Read the model definition and answer for the solid it produces. Units are mm, in the model's axes. Face numbers are marked on the shaded views. Coordinates: 2 decimals unless noted, no trailing zeros. Order: outer loops, then holes, each group sorted by start corner. A loop starts at its lowest first (then second) coordinate and runs counter-clockwise, first axis right, second up. Notation, with made-up numbers: (-31, 59.25) -> (-9, 59.25) arc R14 cw to (-9, 82.25) -> close; hole circle Ø8 at (49.5, 6). An arc over 180 degrees is marked (long way). Answer in a Markdown table with one row per item.
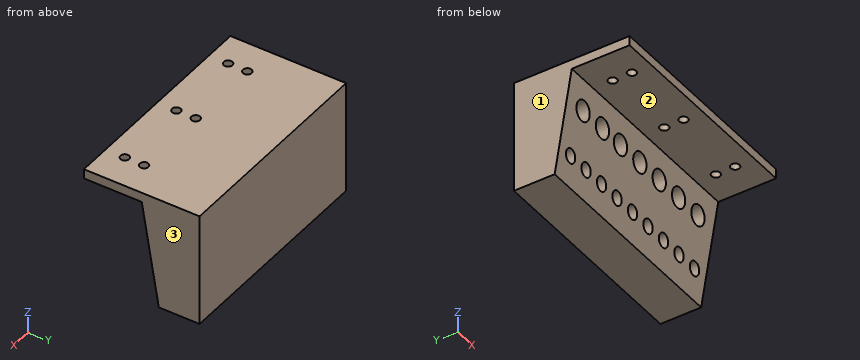
from build123d import *

# Parameters (mm, degrees)
F1_DEPTH = 25
F2_W     = 113.5
F2_H     = 53.5
F3_DEPTH = 5
F5_DEPTH = 133.9
F6_W     = 113.5
F6_H     = 60
F7_DEPTH = 5
F9_DEPTH = 25


with BuildPart() as f1:
    # F0 (on Front) → F1 (new body)
    with BuildSketch(Plane.XZ):
        with BuildLine():
            Line((30.7684078276, 51.75), (-82.7315921724, 51.75))
            Line((-82.7315921724, 51.75), (-82.7315921724, 37.7107225358))
            Line((-82.7315921724, 37.7107225358), (-75.4815921724, 37.7107225358))
            ThreePointArc((-75.4815921724, 37.7107225358), (-70.4815921724, 42.7107225358), (-65.4815921724, 37.7107225358))
            Line((-65.4815921724, 37.7107225358), (-60.4815921724, 37.7107225358))
            ThreePointArc((-60.4815921724, 37.7107225358), (-55.4815921724, 42.7107225358), (-50.4815921724, 37.7107225358))
            Line((-50.4815921724, 37.7107225358), (-46.4815921724, 37.7107225358))
            ThreePointArc((-46.4815921724, 37.7107225358), (-41.4815921724, 42.7107225358), (-36.4815921724, 37.7107225358))
            Line((-36.4815921724, 37.7107225358), (-31.4815921724, 37.7107225358))
            ThreePointArc((-31.4815921724, 37.7107225358), (-26.4815921724, 42.7107225358), (-21.4815921724, 37.7107225358))
            Line((-21.4815921724, 37.7107225358), (-16.4815921724, 37.7107225358))
            ThreePointArc((-16.4815921724, 37.7107225358), (-11.4815921724, 42.7107225358), (-6.4815921724, 37.7107225358))
            Line((-6.4815921724, 37.7107225358), (-1.4815921724, 37.7107225358))
            ThreePointArc((-1.4815921724, 37.7107225358), (3.5184078276, 42.7107225358), (8.5184078276, 37.7107225358))
            Line((8.5184078276, 37.7107225358), (13.5184078276, 37.7107225358))
            ThreePointArc((13.5184078276, 37.7107225358), (18.5184078276, 42.7107225358), (23.5184078276, 37.7107225358))
            Line((23.5184078276, 37.7107225358), (30.7684078276, 37.7107225358))
            Line((30.7684078276, 37.7107225358), (30.7684078276, 51.75))
        make_face()
        with BuildLine():
            Line((-77.4815921724, 12.7484267578), (-82.7315921724, 12.7484267578))
            Line((-82.7315921724, 12.7484267578), (-82.7315921724, -1.75))
            Line((-82.7315921724, -1.75), (30.7684078276, -1.75))
            Line((30.7684078276, -1.75), (30.7684078276, 12.7484267578))
            Line((30.7684078276, 12.7484267578), (25.5184078276, 12.7484267578))
            ThreePointArc((25.5184078276, 12.7484267578), (22.0184078276, 9.2484267578), (18.5184078276, 12.7484267578))
            Line((18.5184078276, 12.7484267578), (13.5184078276, 12.7484267578))
            ThreePointArc((13.5184078276, 12.7484267578), (10.0184078276, 9.2484267578), (6.5184078276, 12.7484267578))
            Line((6.5184078276, 12.7484267578), (1.5184078276, 12.7484267578))
            ThreePointArc((1.5184078276, 12.7484267578), (-1.9815921724, 9.2484267578), (-5.4815921724, 12.7484267578))
            Line((-5.4815921724, 12.7484267578), (-10.4815921724, 12.7484267578))
            ThreePointArc((-10.4815921724, 12.7484267578), (-13.9815921724, 9.2484267578), (-17.4815921724, 12.7484267578))
            Line((-17.4815921724, 12.7484267578), (-22.4815921724, 12.7484267578))
            ThreePointArc((-22.4815921724, 12.7484267578), (-25.9815921724, 9.2484267578), (-29.4815921724, 12.7484267578))
            Line((-29.4815921724, 12.7484267578), (-34.4815921724, 12.7484267578))
            ThreePointArc((-34.4815921724, 12.7484267578), (-37.9815921724, 9.2484267578), (-41.4815921724, 12.7484267578))
            Line((-41.4815921724, 12.7484267578), (-46.4815921724, 12.7484267578))
            ThreePointArc((-46.4815921724, 12.7484267578), (-49.9815921724, 9.2484267578), (-53.4815921724, 12.7484267578))
            Line((-53.4815921724, 12.7484267578), (-58.4815921724, 12.7484267578))
            ThreePointArc((-58.4815921724, 12.7484267578), (-61.9815921724, 9.2484267578), (-65.4815921724, 12.7484267578))
            Line((-65.4815921724, 12.7484267578), (-70.4815921724, 12.7484267578))
            ThreePointArc((-70.4815921724, 12.7484267578), (-73.9815921724, 9.2484267578), (-77.4815921724, 12.7484267578))
        make_face()
        with BuildLine():
            Line((-75.4815921724, 37.7107225358), (-82.7315921724, 37.7107225358))
            Line((-82.7315921724, 37.7107225358), (-82.7315921724, 12.7484267578))
            Line((-82.7315921724, 12.7484267578), (-77.4815921724, 12.7484267578))
            ThreePointArc((-77.4815921724, 12.7484267578), (-73.9815921724, 16.2484267578), (-70.4815921724, 12.7484267578))
            Line((-70.4815921724, 12.7484267578), (-65.4815921724, 12.7484267578))
            ThreePointArc((-65.4815921724, 12.7484267578), (-61.9815921724, 16.2484267578), (-58.4815921724, 12.7484267578))
            Line((-58.4815921724, 12.7484267578), (-53.4815921724, 12.7484267578))
            ThreePointArc((-53.4815921724, 12.7484267578), (-49.9815921724, 16.2484267578), (-46.4815921724, 12.7484267578))
            Line((-46.4815921724, 12.7484267578), (-41.4815921724, 12.7484267578))
            ThreePointArc((-41.4815921724, 12.7484267578), (-37.9815921724, 16.2484267578), (-34.4815921724, 12.7484267578))
            Line((-34.4815921724, 12.7484267578), (-29.4815921724, 12.7484267578))
            ThreePointArc((-29.4815921724, 12.7484267578), (-25.9815921724, 16.2484267578), (-22.4815921724, 12.7484267578))
            Line((-22.4815921724, 12.7484267578), (-17.4815921724, 12.7484267578))
            ThreePointArc((-17.4815921724, 12.7484267578), (-13.9815921724, 16.2484267578), (-10.4815921724, 12.7484267578))
            Line((-10.4815921724, 12.7484267578), (-5.4815921724, 12.7484267578))
            ThreePointArc((-5.4815921724, 12.7484267578), (-1.9815921724, 16.2484267578), (1.5184078276, 12.7484267578))
            Line((1.5184078276, 12.7484267578), (6.5184078276, 12.7484267578))
            ThreePointArc((6.5184078276, 12.7484267578), (10.0184078276, 16.2484267578), (13.5184078276, 12.7484267578))
            Line((13.5184078276, 12.7484267578), (18.5184078276, 12.7484267578))
            ThreePointArc((18.5184078276, 12.7484267578), (22.0184078276, 16.2484267578), (25.5184078276, 12.7484267578))
            Line((25.5184078276, 12.7484267578), (30.7684078276, 12.7484267578))
            Line((30.7684078276, 12.7484267578), (30.7684078276, 37.7107225358))
            Line((30.7684078276, 37.7107225358), (23.5184078276, 37.7107225358))
            ThreePointArc((23.5184078276, 37.7107225358), (18.5184078276, 32.7107225358), (13.5184078276, 37.7107225358))
            Line((13.5184078276, 37.7107225358), (8.5184078276, 37.7107225358))
            ThreePointArc((8.5184078276, 37.7107225358), (3.5184078276, 32.7107225358), (-1.4815921724, 37.7107225358))
            Line((-1.4815921724, 37.7107225358), (-6.4815921724, 37.7107225358))
            ThreePointArc((-6.4815921724, 37.7107225358), (-11.4815921724, 32.7107225358), (-16.4815921724, 37.7107225358))
            Line((-16.4815921724, 37.7107225358), (-21.4815921724, 37.7107225358))
            ThreePointArc((-21.4815921724, 37.7107225358), (-26.4815921724, 32.7107225358), (-31.4815921724, 37.7107225358))
            Line((-31.4815921724, 37.7107225358), (-36.4815921724, 37.7107225358))
            ThreePointArc((-36.4815921724, 37.7107225358), (-41.4815921724, 32.7107225358), (-46.4815921724, 37.7107225358))
            Line((-46.4815921724, 37.7107225358), (-50.4815921724, 37.7107225358))
            ThreePointArc((-50.4815921724, 37.7107225358), (-55.4815921724, 32.7107225358), (-60.4815921724, 37.7107225358))
            Line((-60.4815921724, 37.7107225358), (-65.4815921724, 37.7107225358))
            ThreePointArc((-65.4815921724, 37.7107225358), (-70.4815921724, 32.7107225358), (-75.4815921724, 37.7107225358))
        make_face()
    extrude(amount=F1_DEPTH)

    # F2 (on face) → F3 (join)
    with BuildSketch(Plane(origin=(0, 0, 0), x_dir=(-1, 0, 0), z_dir=(0, 1, 0))):
        with Locations((25.9815921724, 25)):
            Rectangle(F2_W, F2_H)
    extrude(amount=F3_DEPTH)

    # F4 (on face) → F5 (cut)
    with BuildSketch(Plane(origin=(-82.7315921724, 0, 0), x_dir=(0, -1, 0), z_dir=(-1, 0, 0))):
        Polygon((25, -1.75), (25, 51.75), (16.1387622356, -1.75), align=None)
    extrude(amount=-F5_DEPTH, mode=Mode.SUBTRACT)

    # F6 (on face) → F7 (join)
    with BuildSketch(Plane.XY.offset(51.75)):
        with Locations((-25.9815921724, -25)):
            Rectangle(F6_W, F6_H)
    extrude(amount=F7_DEPTH)

    # F8 (on face) → F9 (cut)
    with BuildSketch(Plane(origin=(0, 0, 51.75), x_dir=(1, 0, 0), z_dir=(0, 0, -1))):
        with BuildLine():
            ThreePointArc((-63.7315921724, 45), (-65.9815921724, 47.25), (-68.2315921724, 45))
            Line((-68.2315921724, 45), (-63.7315921724, 45))
        make_face()
        with BuildLine():
            ThreePointArc((16.2684078276, 45), (14.0184078276, 47.25), (11.7684078276, 45))
            Line((11.7684078276, 45), (16.2684078276, 45))
        make_face()
        with BuildLine():
            Line((16.2684078276, 45), (11.7684078276, 45))
            ThreePointArc((11.7684078276, 45), (14.0184078276, 42.75), (16.2684078276, 45))
        make_face()
        with BuildLine():
            ThreePointArc((-23.7315921724, 45), (-25.9815921724, 47.25), (-28.2315921724, 45))
            Line((-28.2315921724, 45), (-23.7315921724, 45))
        make_face()
        with BuildLine():
            Line((-23.7315921724, 45), (-28.2315921724, 45))
            ThreePointArc((-28.2315921724, 45), (-25.9815921724, 42.75), (-23.7315921724, 45))
        make_face()
        with BuildLine():
            Line((-63.7315921724, 45), (-68.2315921724, 45))
            ThreePointArc((-68.2315921724, 45), (-65.9815921724, 42.75), (-63.7315921724, 45))
        make_face()
        with BuildLine():
            ThreePointArc((-63.7315921724, 35), (-65.9815921724, 37.25), (-68.2315921724, 35))
            Line((-68.2315921724, 35), (-63.7315921724, 35))
        make_face()
        with BuildLine():
            ThreePointArc((16.2684078276, 35), (14.0184078276, 37.25), (11.7684078276, 35))
            Line((11.7684078276, 35), (16.2684078276, 35))
        make_face()
        with BuildLine():
            Line((16.2684078276, 35), (11.7684078276, 35))
            ThreePointArc((11.7684078276, 35), (14.0184078276, 32.75), (16.2684078276, 35))
        make_face()
        with BuildLine():
            ThreePointArc((-23.7315921724, 35), (-25.9815921724, 37.25), (-28.2315921724, 35))
            Line((-28.2315921724, 35), (-23.7315921724, 35))
        make_face()
        with BuildLine():
            Line((-23.7315921724, 35), (-28.2315921724, 35))
            ThreePointArc((-28.2315921724, 35), (-25.9815921724, 32.75), (-23.7315921724, 35))
        make_face()
        with BuildLine():
            Line((-63.7315921724, 35), (-68.2315921724, 35))
            ThreePointArc((-68.2315921724, 35), (-65.9815921724, 32.75), (-63.7315921724, 35))
        make_face()
    extrude(amount=-F9_DEPTH, mode=Mode.SUBTRACT)


solid = f1.part
Q1. The part is cut by section A-A (y = -45). Write down the section's boundary in (x, z).
Outcome:
| item | result |
|---|---|
| outline | (-82.73, 51.75) -> (-68.23, 51.75) -> (-68.23, 56.75) -> (-82.73, 56.75) -> close; (-63.73, 51.75) -> (-28.23, 51.75) -> (-28.23, 56.75) -> (-63.73, 56.75) -> close; (-23.73, 51.75) -> (11.77, 51.75) -> (11.77, 56.75) -> (-23.73, 56.75) -> close; (16.27, 51.75) -> (30.77, 51.75) -> (30.77, 56.75) -> (16.27, 56.75) -> close |
Q2. The part is cut by section B-B (y = -2). Give the number of separate pieces and of enclosed holes in the cut face, then the cut area to 3 significant figures.
Outcome:
| item | result |
|---|---|
| separate pieces | 1 |
| enclosed holes | 16 |
| area | 5,740 mm² |
Q3. For a pull along X with two mould halves and no side action, classify the marked faces 1, 2 and 3 as pulls with the +X half, pulls with the -X half, needs draft (parallel to the pull), parting line crosses it, or undercut.
Outcome:
| item | result |
|---|---|
| face 1 | pulls with the -X half |
| face 2 | needs draft |
| face 3 | pulls with the +X half |
Q4. Given pin 1 (2 mm diameter, centred on x = -62, z = 13.5, fed in from -Y); pin 2 (11 mm diameter, centred on x = 10.02, z = 12.75, fed in from -Y); pin 3 (11.5 mm diameter, centred on x = 3.52, z = 37.71, fed in from -Y), each flat-ended and moving along its own axis, determine where each tip first touches the part or whether it passes through.
Outcome:
| item | result |
|---|---|
| pin 1 | y = 0 |
| pin 2 | y = -19.45 |
| pin 3 | y = -23.63 |
Q5. Consider line 1 (Z direction, x = 19.5, y = -8); line 2 (Z direction, x = 20, y = -4.5); line 3 (Y direction, x = 21, z = 40). Determine where each line is inside the solid, lowest interval first.
Outcome:
| item | result |
|---|---|
| line 1 | -1.75 to 10.32, 15.18 to 32.81, 42.61 to 56.75 |
| line 2 | -1.75 to 9.89, 15.61 to 32.94, 42.49 to 56.75 |
| line 3 | 0 to 5 |
Q6. The part is cut by section D-D (z = 7.5). Write down the section's boundary in (x, y), then the cut area to 3 significant figures.
Outcome:
| item | result |
|---|---|
| outline | (-82.73, -17.67) -> (30.77, -17.67) -> (30.77, 5) -> (-82.73, 5) -> close |
| area | 2,570 mm² |
